CAD build for the part. Positions are in the model's coordinates, mm. Face numbers are marked on the shaded views. Give positions to 0.01 mm unless a question says otherwise; leave off trailing zeros. Order: outer loops, then holes, each group sorted by start corner. A loop starts at its lowest first (then second) coordinate and runs counter-clockwise, first axis right, second up.
Item 1: Wall check: L1, parallel to Z at x = -6, y = -53 (3 decimals); L2, parallel to X at y = -11, z = 6.25; L3, parallel to X at y = -65, z = 11.75. Give the ranges that are in metal, low to high.
Item 2: Band-saw the part on D-D on y = -32. Give the cut face in (x, z) (3 decimals), plus the area to 3 significant figures.
Item 3: Flat gauge pins, fed straight in: P1, Ø3.5, axis at y = -23, z = 1, coming from the -X side; P2, Ø4, axis at x = -97, y = -41.5, coming from the -Z side; P3, Ø4, axis at x = -12.7, y = -6.35, coming from the +Z side (3 decimals); P4, Ø6, axis at y = -55.5, z = 9, coming from the -X side. Where does each tip first touch, or does it go through?
Item 4: Band-saw the part on B-B on y = -6.35. Give the cut face in (x, z) (3 decimals).
Item 5: Two-plate mould, pull along X, no slides. Class the marked faces 1, 2, 3 and 4: released by +X, released by -X, zero draft, split by the parting line, or undercut.
Item 6: Band-saw the part on A-A on y = -16. Give the cut face in (x, z) (3 decimals).
Item 7: Band-saw the part on C-C on x = -95. Give the cut face in (y, z) (3 decimals), plus the area to 3 significant figures.
```python
from build123d import *

# Parameters (mm, degrees)
SKETCH1_W           = 114.3
SKETCH1_H           = 76.2
BOSS_EXTRUDE1_DEPTH = 3.175
BOSS_EXTRUDE2_DEPTH = 76.2
SKETCH3_R           = 1.778
CUT_EXTRUDE1_DEPTH  = 203.2
CUT_EXTRUDE2_DEPTH  = 3.175
LPATTERN1_COUNT     = 3
LPATTERN1_PITCH     = 31.75
SKETCH5_R           = 1.778
CUT_EXTRUDE3_DEPTH  = 3.175
SKETCH6_R           = 1.778
CUT_EXTRUDE4_DEPTH  = 3.175


with BuildPart() as part:
    # Sketch1 → Boss-Extrude1 (new body)
    with BuildSketch(Plane.XY):
        with Locations((-57.15, -38.1)):
            Rectangle(SKETCH1_W, SKETCH1_H)
    extrude(amount=BOSS_EXTRUDE1_DEPTH)

    # Sketch2 → Boss-Extrude2 (add)
    with BuildSketch(Plane.XZ.offset(76.2)):
        Polygon((-114.3, 3.175), (-117.087804878, 15.565243902), (-120.185365854, 14.868292683), (-116.84, 0), (-114.3, 0), align=None)
        Polygon((0, 3.175), (0, 0), (13.087195122, 2.865243902), (12.390243902, 5.962804878), align=None)
    extrude(amount=-BOSS_EXTRUDE2_DEPTH)

    # Sketch3 → Cut-Extrude1 (cut)
    with BuildSketch(Plane(origin=(-108.112433076, 0, -24.325297442), x_dir=(0.219512195, 0, -0.975609756), z_dir=(0.975609756, 0, 0.219512195))):
        with Locations((-34.537804878, -12.7)):
            Circle(SKETCH3_R)
        with Locations((-34.537804878, -63.5)):
            Circle(SKETCH3_R)
    extrude(amount=-CUT_EXTRUDE1_DEPTH, mode=Mode.SUBTRACT)

    # Sketch4 → Cut-Extrude2 (cut)
    with BuildSketch(Plane.XY.offset(3.175)):
        Polygon((-101.6, -63.5), (-101.6, -38.1), (-76.2, -50.8), align=None)
        Polygon((-101.6, -25.4), (-76.2, -38.1), (-76.2, -12.7), align=None)
    cut_extrude2 = extrude(amount=-CUT_EXTRUDE2_DEPTH, mode=Mode.SUBTRACT)

    # LPattern1: Cut-Extrude2 ×3
    with Locations(*[(i * LPATTERN1_PITCH, 0, 0) for i in range(1, LPATTERN1_COUNT)]):
        add(cut_extrude2, mode=Mode.SUBTRACT)

    # Sketch5 → Cut-Extrude3 (cut)
    with BuildSketch(Plane.XY.offset(3.175)):
        with Locations((-101.6, -69.85)):
            Circle(SKETCH5_R)
        with Locations((-12.7, -69.85)):
            Circle(SKETCH5_R)
        with Locations((-12.7, -6.35)):
            Circle(SKETCH5_R)
        with Locations((-101.6, -6.35)):
            Circle(SKETCH5_R)
    extrude(amount=-CUT_EXTRUDE3_DEPTH, mode=Mode.SUBTRACT)

    # Sketch6 → Cut-Extrude4 (cut)
    with BuildSketch(Plane(origin=(-0.679952409, 0, 3.022010708), x_dir=(0.975609756, 0, 0.219512195), z_dir=(-0.219512195, 0, 0.975609756))):
        with Locations((7.04695122, -63.5)):
            Circle(SKETCH6_R)
        with Locations((7.04695122, -12.7)):
            Circle(SKETCH6_R)
    extrude(amount=-CUT_EXTRUDE4_DEPTH, mode=Mode.SUBTRACT)


solid = part.part
```
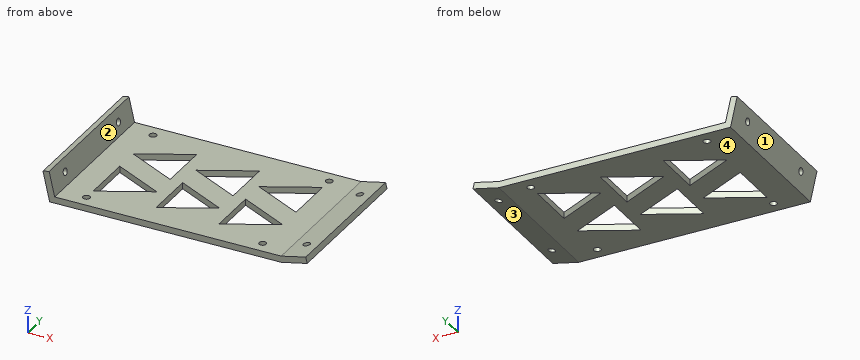
The answers:
1. L1: z = 0 to 3.175
1. L2: x = -118.25 to -114.99
1. L3: x = -119.48 to -116.23
2. outline: (-120.185, 14.868) - (-116.84, 0) - (-88.4, 0) - (-88.4, 3.175) - (-114.3, 3.175) - (-117.088, 15.565) - close; (-76.2, 0) - (-56.65, 0) - (-56.65, 3.175) - (-76.2, 3.175) - close; (-44.45, 0) - (-24.9, 0) - (-24.9, 3.175) - (-44.45, 3.175) - close; (-12.7, 0) - (0, 0) - (13.087, 2.865) - (12.39, 5.963) - (0, 3.175) - (-12.7, 3.175) - close
2. area: 336 mm2
3. P1: stops at x = -117.46
3. P2: stops at z = 0
3. P3: stops at z = 3.175
3. P4: stops at x = -119.54
4. outline: (-120.185, 14.868) - (-116.84, 0) - (-103.378, 0) - (-103.378, 3.175) - (-114.3, 3.175) - (-117.088, 15.565) - close; (-99.822, 0) - (-14.478, 0) - (-14.478, 3.175) - (-99.822, 3.175) - close; (-10.922, 0) - (0, 0) - (13.087, 2.865) - (12.39, 5.963) - (0, 3.175) - (-10.922, 3.175) - close
5. face 1: released by -X
5. face 2: undercut
5. face 3: released by +X
5. face 4: zero draft
6. outline: (-120.185, 14.868) - (-116.84, 0) - (-82.8, 0) - (-82.8, 3.175) - (-114.3, 3.175) - (-117.088, 15.565) - close; (-76.2, 0) - (-51.05, 0) - (-51.05, 3.175) - (-76.2, 3.175) - close; (-44.45, 0) - (-19.3, 0) - (-19.3, 3.175) - (-44.45, 3.175) - close; (-12.7, 0) - (0, 0) - (13.087, 2.865) - (12.39, 5.963) - (0, 3.175) - (-12.7, 3.175) - close
7. outline: (-76.2, 0) - (-60.2, 0) - (-60.2, 3.175) - (-76.2, 3.175) - close; (-41.4, 0) - (-28.7, 0) - (-28.7, 3.175) - (-41.4, 3.175) - close; (-22.1, 0) - (0, 0) - (0, 3.175) - (-22.1, 3.175) - close
7. area: 161 mm2
